```python
from build123d import *

# Parameters (mm, degrees)
F0_W      = 380
F0_H      = 380
F1_DEPTH  = 350
F2_W      = 342
F2_H      = 322
F3_DEPTH  = 342
F4_W      = 40
F4_H      = 40
F5_DEPTH  = 150
F6_W      = 40
F6_H      = 40
F7_DEPTH  = 150
F8_W      = 40
F8_H      = 40
F9_DEPTH  = 150
F10_W     = 40
F10_H     = 40
F11_DEPTH = 150


with BuildPart() as f1:
    # F0 (on Top) → F1 (new body)
    with BuildSketch(Plane.XY):
        Rectangle(F0_W, F0_H)
    extrude(amount=F1_DEPTH)

    # F2 (on face) → F3 (cut)
    with BuildSketch(Plane.XZ.offset(190)):
        with Locations((0, 175)):
            Rectangle(F2_W, F2_H)
    extrude(amount=-F3_DEPTH, mode=Mode.SUBTRACT)

    # F4 (on face) → F5 (join)
    with BuildSketch(Plane(origin=(0, 0, 0), x_dir=(1, 0, 0), z_dir=(0, 0, -1))):
        with Locations((-170, 170)):
            Rectangle(F4_W, F4_H)
    extrude(amount=F5_DEPTH)

    # F6 (on face) → F7 (join)
    with BuildSketch(Plane(origin=(0, 0, 0), x_dir=(1, 0, 0), z_dir=(0, 0, -1))):
        with Locations((170, 170)):
            Rectangle(F6_W, F6_H)
    extrude(amount=F7_DEPTH)

    # F8 (on face) → F9 (join)
    with BuildSketch(Plane(origin=(0, 0, 0), x_dir=(1, 0, 0), z_dir=(0, 0, -1))):
        with Locations((-170, -170)):
            Rectangle(F8_W, F8_H)
    extrude(amount=F9_DEPTH)

    # F10 (on face) → F11 (join)
    with BuildSketch(Plane(origin=(0, 0, 0), x_dir=(1, 0, 0), z_dir=(0, 0, -1))):
        with Locations((170, -170)):
            Rectangle(F10_W, F10_H)
    extrude(amount=F11_DEPTH)


solid = f1.part
```
Here's how the part is built. I have some questions about the finished solid (model axes, mm). A direction names the side the tool comes from. Round coordinates to 2 decimals unless told otherwise and drop trailing zeros. Loops run counter-clockwise (first coordinate to the right, second up) from the corner with the lowest first, then second, coordinate; pieces in that order, holes last.
1. Will these pins go through, and if not, where does the flat tip stop? pin 1 (4 mm diameter, centred on x = -101, y = 91.5, fed in from -Z); pin 2 (10 mm diameter, centred on x = 62.5, z = 136.5, fed in from -Y).
Answers:
pin 1: stops at z = 0
pin 2: stops at y = 152
2. If I drill on probe 1 along Z at (x, y) = (20, -46); probe 2 along X at (y, z) = (-4, 128.5); probe 3 along Y at (x, z) = (135, 287), over which ranges is the centre line in solid material (lowest first)?
Answers:
probe 1: z = 0 to 14, 336 to 350
probe 2: x = -190 to -171, 171 to 190
probe 3: y = 152 to 190
3. Suppose I cut it at A-A, the plane z = -114.5. Please give me the cut outline in (x, y).
Answers:
outline: (-190, -190) - (-150, -190) - (-150, -150) - (-190, -150) - close; (-190, 150) - (-150, 150) - (-150, 190) - (-190, 190) - close; (150, -190) - (190, -190) - (190, -150) - (150, -150) - close; (150, 150) - (190, 150) - (190, 190) - (150, 190) - close
4. For faces 4 (the face through (171, -21, 173)), 5 (the face through (170, -150, -74)), 6 (the face through (150, -170, -74)), which set-ups out of +Z, -Z, +X, -X, +Y, -Y let a thin tool reach every point of the face, with its end or its side?
Answers:
face 4: -Y
face 5: -Z, +X, -X
face 6: -Z, +Y, -Y
5. Thinking about a two-plate mould opening in X: for faces 1 (the face through (-3, 3, 0)), 2 (the face through (170, -170, -150)), 3 (the face through (190, 3, 159)), which applies, released by +X, released by -X, zero draft, split by the parting line, or undercut?
Answers:
face 1: undercut
face 2: zero draft
face 3: released by +X
6. Suppose I cut it at B-B, the plane y = 126. Please give me the cut outline in (x, z), and give its area (3 significant figures).
Answers:
outline: (-190, 0) - (190, 0) - (190, 350) - (-190, 350) - close; hole (-171, 14) - (171, 14) - (171, 336) - (-171, 336) - close
area: 22,900 mm2
7. Suppose I cut it at D-D, the plane z = 79.5. Please give me the cut outline in (x, y).
Answers:
outline: (-190, -190) - (-171, -190) - (-171, 152) - (171, 152) - (171, -190) - (190, -190) - (190, 190) - (-190, 190) - close
8. Suppose I cut it at C-C, the plane x = 37. Please give me the cut outline in (y, z).
Answers:
outline: (-190, 0) - (190, 0) - (190, 350) - (-190, 350) - (-190, 336) - (152, 336) - (152, 14) - (-190, 14) - close
